CAD build for the part. Positions are in the model's coordinates, mm. A direction names the side the tool comes from. Coordinates: 2 decimals unless noted, no trailing zeros. Write each loop counter-clockwise with the first axis right and the second up, starting at its lowest first coordinate (ties: lowest second). Pieces come first, ordered by that corner, then holes.
```python
from build123d import *

# Parameters (mm, degrees)
BOSS_EXTRUDE1_DEPTH     = 119
CUT_EXTRUDE1_DEPTH      = 117
CUT_EXTRUDE2_DEPTH      = 121.479251326
SKETCH5_W               = 10
SKETCH5_H               = 2
CUT_EXTRUDE4_DEPTH      = 123.172009888
CUT_EXTRUDE5_DEPTH      = 121.030204532
CUT_EXTRUDE5_DEPTH_BACK = 121.030204532
SKETCH7_W               = 6
SKETCH7_H               = 2.5
BOSS_EXTRUDE2_DEPTH     = 2.5
SKETCH10_R              = 1
CUT_EXTRUDE6_DEPTH      = 6


with BuildPart() as part:
    # Sketch1 → Boss-Extrude1 (new body)
    with BuildSketch(Plane.XY):
        with BuildLine():
            Line((-6, 12.5), (6, 12.5))
            Line((6, 12.5), (6, -12.5))
            ThreePointArc((6, -12.5), (5.414213562, -13.914213562), (4, -14.5))
            Line((4, -14.5), (-4, -14.5))
            ThreePointArc((-4, -14.5), (-5.414213562, -13.914213562), (-6, -12.5))
            Line((-6, -12.5), (-6, 12.5))
        make_face()
    extrude(amount=BOSS_EXTRUDE1_DEPTH)

    # Sketch2 → Cut-Extrude1 (cut)
    with BuildSketch(Plane(origin=(0, 0, 0), x_dir=(-1, 0, 0), z_dir=(0, 0, -1))):
        with BuildLine():
            Line((-5, -8.3), (-5, 11.5))
            Line((-5, 11.5), (5, 11.5))
            Line((5, 11.5), (5, -8.3))
            ThreePointArc((5, -8.3), (0, -13.3), (-5, -8.3))
        make_face()
    extrude(amount=-CUT_EXTRUDE1_DEPTH, mode=Mode.SUBTRACT)

    # Sketch3 → Cut-Extrude2 (cut, through all)
    with BuildSketch(Plane(origin=(6, 0, 0), x_dir=(0, 0, -1), z_dir=(1, 0, 0))):
        with BuildLine():
            Line((-8.499997834, -5), (-110.499997834, -5))
            ThreePointArc((-110.499997834, -5), (-115.500002166, -2.166e-06), (-110.500002166, 5))
            Line((-110.500002166, 5), (-8.500002166, 5))
            ThreePointArc((-8.500002166, 5), (-3.500002166, 2.166e-06), (-8.499997834, -5))
        make_face()
    extrude(amount=-CUT_EXTRUDE2_DEPTH, mode=Mode.SUBTRACT)

    # Sketch5 → Cut-Extrude4 (cut, through all)
    with BuildSketch(Plane(origin=(0, 12.5, 0), x_dir=(1, 0, 0), z_dir=(0, 1, 0))):
        Rectangle(SKETCH5_W, SKETCH5_H)
    extrude(amount=-CUT_EXTRUDE4_DEPTH, mode=Mode.SUBTRACT)

    # Sketch6 → Cut-Extrude5 (cut, two sides: drawn at the far end of the back side and taken through both)
    with BuildSketch(Plane(origin=(0, 0, 0), x_dir=(0, 0, -1), z_dir=(1, 0, 0)).offset(-CUT_EXTRUDE5_DEPTH_BACK)):
        Polygon((0, 0), (-10, -14.5), (0, -14.5), align=None)
    extrude(amount=CUT_EXTRUDE5_DEPTH + CUT_EXTRUDE5_DEPTH_BACK, mode=Mode.SUBTRACT)

    # Sketch7 → Boss-Extrude2 (add)
    with BuildSketch(Plane(origin=(0, 0, 117), x_dir=(-1, 0, 0), z_dir=(0, 0, -1))):
        with Locations((0, -11)):
            Rectangle(SKETCH7_W, SKETCH7_H)
    extrude(amount=BOSS_EXTRUDE2_DEPTH)

    # Sketch10 → Cut-Extrude6 (cut)
    with BuildSketch(Plane.ZY.offset(3)):
        with Locations((115.75, -11)):
            Circle(SKETCH10_R)
    extrude(amount=-CUT_EXTRUDE6_DEPTH, mode=Mode.SUBTRACT)


solid = part.part
```
Item 1: Saw through at A-A, the plane z = 106. Write the cut outline in (x, y), and give its area (3 significant figures).
Item 2: Flat gauge pins, fed straight in: pin 1 Ø0.8 at (x, y) = (-0.5, 12) entering from -Z; pin 2 Ø3 at (x, y) = (0.5, -5) entering from -Z; pin 3 Ø0.5 at (x, z) = (-5.5, 34.5) entering from -Y. Where does each tip first touch, or does it go through?
Item 3: Wall check: line 1 along Y through (x, z) = (0, 112.5); line 2 along X through (y, z) = (10, 46); line 3 along Y through (x, z) = (-0.85, 115.75). Give the ranges that are in metal, low to high.
Item 4: Two-plate mould, pull along Y, no slides. Class faces 4 (the cylindrical face through (-0.04, -10.96, 114.75)), 5 (the cylindrical face through (5.43, -13.9, 63.04)), 6 (the flat face through (0, -1, 119)), 7 (the flat face through (0, 12.5, 59)): +Y half, -Y half, draft (parallel to the pull), parting line (faces both ways), or undercut.
Item 5: Which spindle directions (+Z, -Z, +X, -X, +Y, -Y) get a long thin tool onto all of the face, cutting with end or side? Do faces 1 (the flat face through (0, -14.5, 64)), 2 (the flat face through (-5, 7, 59)), 3 (the cylindrical face through (5.5, 0.1, 3.5)). Say none if no direction does.
Item 6: Saw through at C-C, the plane y = -11. Write the cut outline in (x, z).
Item 7: Saw through at B-B, the plane x = 0. Write the cut outline in (y, z).
Working result:
1. outline: (-6, -12.5) arc R2 ccw to (-4, -14.5) - (4, -14.5) arc R2 ccw to (6, -12.5) - (6, -5) - (5, -5) - (5, -8.3) arc R5 cw to (-5, -8.3) - (-5, -5) - (-6, -5) - close; (-6, 5) - (-5, 5) - (-5, 11.5) - (5, 11.5) - (5, 5) - (6, 5) - (6, 12.5) - (-6, 12.5) - close
1. area: 65.0 mm2
2. pin 1: stops at z = 1
2. pin 2: stops at z = 117
2. pin 3: stops at y = -14.06
3. line 1: y = -14.5 to -13.3, 11.5 to 12.5
3. line 2: x = -6 to -5, 5 to 6
3. line 3: y = -14.5 to -13.23, -12.25 to -12, -10 to -9.75, 11.5 to 12.5
4. face 4: undercut
4. face 5: -Y half
4. face 6: draft
4. face 7: +Y half
5. face 1: +Z, -Z, +X, -X, -Y
5. face 2: -Z
5. face 3: +X, -X
6. outline: (-6, 7.59) - (-4.21, 7.59) - (-4.21, 117) - (-3, 117) - (-3, 116.75) - (3, 116.75) - (3, 117) - (4.21, 117) - (4.21, 7.59) - (6, 7.59) - (6, 119) - (-6, 119) - close; (-3, 114.5) - (3, 114.5) - (3, 114.75) - (-3, 114.75) - close
7. outline: (-14.5, 10) - (-13.3, 9.17) - (-13.3, 117) - (-12.25, 117) - (-12.25, 114.5) - (-9.75, 114.5) - (-9.75, 117) - (11.5, 117) - (11.5, 1) - (12.5, 1) - (12.5, 119) - (-14.5, 119) - close; hole circle Ø2 at (-11, 115.75)
